```python
from build123d import *

# Parameters (mm, degrees)
F1_DEPTH = 3


with BuildPart() as f1:
    # F0 (on Front) → F1 (new body)
    with BuildSketch(Plane.XZ):
        Polygon((152.0495, -30.5), (167.2495, -30.5), (167.2495, -27.5), (167.2495, -20.33), (164.2495, -20.33), (164.2495, -10.164), (167.2495, -10.164), (167.2495, 0.002), (164.2495, 0.002), (164.2495, 10.168), (167.2495, 10.168), (167.2495, 20.334), (164.2495, 20.334), (164.2495, 30.5), (-164.2495, 30.5), (-164.2495, 20.334), (-167.2495, 20.334), (-167.2495, 10.168), (-164.2495, 10.168), (-164.2495, 0.002), (-167.2495, 0.002), (-167.2495, -10.164), (-164.2495, -10.164), (-164.2495, -20.33), (-167.2495, -20.33), (-167.2495, -27.5), (-152.0495, -27.5), (-152.0495, -30.5), (-136.8495, -30.5), (-136.8495, -27.5), (-121.6495, -27.5), (-121.6495, -30.5), (-106.4495, -30.5), (-106.4495, -27.5), (-91.2495, -27.5), (-91.2495, -30.5), (-76.0495, -30.5), (-76.0495, -27.5), (-60.8495, -27.5), (-60.8495, -30.5), (-45.6495, -30.5), (-45.6495, -27.5), (-30.4495, -27.5), (-30.4495, -30.5), (-15.2495, -30.5), (-15.2495, -27.5), (-0.0495, -27.5), (0.0495, -27.5), (0.0495, -30.5), (15.2495, -30.5), (15.2495, -27.5), (30.4495, -27.5), (30.4495, -30.5), (45.6495, -30.5), (45.6495, -27.5), (60.8495, -27.5), (60.8495, -30.5), (76.0495, -30.5), (76.0495, -27.5), (91.2495, -27.5), (91.2495, -30.5), (106.4495, -30.5), (106.4495, -27.5), (121.6495, -27.5), (121.6495, -30.5), (136.8495, -30.5), (136.8495, -27.5), (152.0495, -27.5), align=None)
    extrude(amount=F1_DEPTH)


solid = f1.part
```
The model under review builds one solid part; all positions refer to its coordinate system, in mm. Round coordinates to 2 decimals unless told otherwise and drop trailing zeros. Order: outer loops, then holes, each group sorted by start corner. A loop starts at its lowest first (then second) coordinate and runs counter-clockwise, first axis right, second up.
Item 1: To check wall thickness, follow probe 1 along Z at (x, y) = (-153, -0.75); probe 2 along X at (y, z) = (-0.5, 4). State the ranges of each line that lie inside material, in increasing order.
Working result:
probe 1: z = -27.5 to 30.5
probe 2: x = -164.25 to 164.25
Item 2: For pin 1 (1.5 mm diameter, centred on x = -67, y = -2, fed in from -Z); pin 2 (0.9 mm diameter, centred on y = -1.5, z = 7, fed in from -X); pin 3 (1.5 mm diameter, centred on y = -1, z = -29.5, fed in from -X), all flat-tipped, find the tip position at first contact; note any pin that passes through.
Working result:
pin 1: stops at z = -27.5
pin 2: stops at x = -164.25
pin 3: stops at x = -152.05
Item 3: Add section A-A, the plane z = 25. State the section outline as (x, y) points, and give its area (3 significant figures).
Working result:
outline: (-164.25, -3) - (164.25, -3) - (164.25, 0) - (-164.25, 0) - close
area: 985 mm2
